Autodesk Inventor part; units mm, degrees
ref_plane "YZ Plane" through (0, 0, 0) normal (1, 0, 0) x (0, 1, 0)
ref_plane "XZ Plane" through (0, 0, 0) normal (0, 1, 0) x (-1, 0, 0)
ref_plane "XY Plane" through (0, 0, 0) normal (0, 0, 1) x (1, 0, 0)
sketch "Sketch1" plane through (0, 0, 0) normal (0, 1, 0) x (-1, 0, 0)
  line L0 (0, 0) -> (-40, 0)
  line L1 (-40, 0) -> (-160, 10)
  line L2 (-160, 10) -> (-160, 15)
  line L3 (-160, 15) -> (0, 15)
  line L4 (0, 15) -> (0, 0)
  point P0 (-160, 12.5)
  dimension "d0" = 15
  dimension "d1" = 40
  dimension "d2" = 5
  dimension "d3" = 120
extrude "Extrusion1" add sketch "Sketch1" along normal blind 16
sketch "Sketch2" plane through (0, 0, 15) normal (0, 0, 1) x (1, 0, 0)
  circle A0 centre (152.5, 8) radius 2.286
  circle A1 centre (47.5, 8) radius 2.286
  line L0 (160, 0) -> (160, 16)
  point P0 (0, 0)
  point P1 (160, 8)
  dimension "d6" = 4.572
  dimension "d7" = 7.5
  dimension "d8" = 105
extrude "Extrusion2" cut sketch "Sketch2" against normal blind 20
sketch "Sketch3" plane through (40, 0, 0) normal (0, 0, -1) x (-1, 0, 0)
  circle A0 centre (-112.5, 8) radius 2.286
  circle A1 centre (-112.5, 8) radius 6
  circle A2 centre (-7.5, 8) radius 2.286
  circle A3 centre (-7.5, 8) radius 6
  point P0 (40, 0)
  dimension "d11" = 12
extrude "Extrusion3" cut sketch "Sketch3" against normal up to surface (10 mm away)
sketch "Sketch4" plane through (40, 0, 0) normal (0, 0, -1) x (-1, 0, 0)
  line L0 (40, 0) -> (40, 16)
  line L1 (40, 0) -> (40, 16)
  line L2 (40, 16) -> (40, 26.5)
  line L3 (40, 26.5) -> (0, 26.5)
  line L4 (0, 26.5) -> (0, 16)
  line L5 (0, 0) -> (0, 16)
  line L6 (0, 0) -> (40, 0)
  line L7 (40, 0) -> (40, 16)
  line L8 (0, 16) -> (40, 16)
  point P0 (40, 8)
  dimension "d14" = 18.5
extrude "Extrusion4" add sketch "Sketch4" against normal up to surface (15 mm away) contours L8 L4 L3 L2
sketch "Sketch5" plane through (40, 0, 0) normal (0, 0, -1) x (-1, 0, 0)
  line L0 (40, 0) -> (-120, 0)
  line L1 (2, 0) -> (2, 13.8)
  line L2 (2, 13.8) -> (40, 13.8)
  line L3 (40, 0) -> (40, 26.5)
  line L4 (40, 26.5) -> (0, 26.5)
  line L5 (0, 26.5) -> (0, 16)
  dimension "d17" = 12.7
  dimension "d18" = 2
extrude "Extrusion5" cut sketch "Sketch5" against normal through all
sketch "Sketch6" plane through (40, 0, 15) normal (0, 0, -1) x (-1, 0, 0)
  line L0 (40, 13.8) -> (40, 26.5)
  line L1 (2, 13.8) -> (2, 0)
  line L2 (40, 13.8) -> (2, 0)
  line L3 (2, 13.8) -> (40, 13.8)
  point P0 (40, 0)
extrude "Extrusion6" add sketch "Sketch6" along normal blind 3
chamfer "Chamfer1" distance 3 angle 45 3 edges at (38, 6.9, 12) (38, 13.8, 6) (19, 13.8, 12)
sketch "Sketch7" plane through (160, 0, 15) normal (0, 0, 1) x (1, 0, 0)
  line L0 (-120, 26.5) -> (-120, 16)
  line L1 (-120, 26.5) -> (-85, 16)
  line L2 (-120, 16) -> (0, 16)
  point P0 (-160, 0)
  dimension "d29" = 35
extrude "Extrusion7" add sketch "Sketch7" against normal up to surface surface through (160, 0, 10) normal (0.0830455, 0, -0.9965458)
sketch "Sketch9" plane through (160, 0, 15) normal (0, 0, 1) x (1, 0, 0)
  circle A0 centre (-140, 21.15) radius 2.794
  circle A1 centre (-155, 21.15) radius 2.794
  line L0 (-160, 13.8) -> (-160, 26.5)
  point P0 (-160, 0)
  point P1 (-160, 15.8)
  point P2 (-160, 21.15)
  dimension "d32" = 5.588
  dimension "d33" = 15
  dimension "d34" = 5
extrude "Extrusion8" cut sketch "Sketch9" against normal through all
properties part number "Fan_side_mount"
For this review, take the finished solid that the model builds, in its own axes (mm). A direction names the side the tool comes from. Coordinates: 2 decimals unless noted, no trailing zeros. Order: outer loops, then holes, each group sorted by start corner. A loop starts at its lowest first (then second) coordinate and runs counter-clockwise, first axis right, second up. Notation, with made-up numbers: (-12.5, 31) -> (42.5, 31) arc R24 ccw to (42.5, 46) -> close; hole circle Ø9 at (59, 7). An arc over 180 degrees is marked (long way). Return JSON: item names as keys, results as strings.
1. We need section C-C on x = 70.5. Write out the cut boundary in (y, z).
Answer block:
{"outline": "(0, 2.54) -> (17.35, 2.54) -> (17.35, 15) -> (0, 15) -> close"}
2. The part is to be moulded in two halves that separate along Y. For faces 1 (the cylindrical face through (150.216, 8.101, 12.535)), 2 (the flat face through (86, 0, 9)), 3 (the flat face through (37, 5, 10)), 4 (the cylindrical face through (146.96, 5.7, 9.55)), say which applies: +Y half, -Y half, draft (parallel to the pull), parting line (faces both ways), or undercut.
Answer block:
{"face 1": "undercut", "face 2": "-Y half", "face 3": "draft", "face 4": "undercut"}
3. For line 1 (Y direction, x = 152.5, z = 11.2); line 2 (Y direction, x = 86, z = 10); line 3 (Y direction, x = 5, z = 12.25), list the stretches that pass through material, from the lowest coordinate up. Write a range as from..to.
Answer block:
{"line 1": "0..5.71, 10.29..16", "line 2": "0..16", "line 3": "11.98..18.36, 23.94..26.5"}
4. We need section D-D on y = 8. Write out the cut boundary in (x, z) (3 decimals), and give its area (3 significant figures).
Answer block:
{"outline": "(15.971, 12) -> (35, 12) -> (38, 9) -> (38, 0) -> (40, 0) -> (41.5, 0.125) -> (41.5, 10) -> (45.214, 10) -> (45.214, 15) -> (15.971, 15) -> close; (49.786, 10) -> (53.5, 10) -> (53.5, 1.125) -> (146.5, 8.875) -> (146.5, 10) -> (150.214, 10) -> (150.214, 15) -> (49.786, 15) -> close; (154.786, 10) -> (158.5, 10) -> (158.5, 9.875) -> (160, 10) -> (160, 15) -> (154.786, 15) -> close", "area": "1,130 mm²"}
5. We need section A-A on x = 5. Write out the cut boundary in (y, z), and give its area (3 significant figures).
Answer block:
{"outline": "(11.98, 10.82) -> (13.8, 9) -> (13.8, 0) -> (18.36, 0) -> (18.36, 15) -> (11.98, 15) -> close; (23.94, 0) -> (26.5, 0) -> (26.5, 15) -> (23.94, 15) -> close", "area": "116 mm²"}
6. Machinability: for faces 5 (the cylindrical face through (41.96, 5.7, 4.99)), 6 (the flat face through (25, 7, 12)), 7 (the flat face through (57.255, 21.323, 7.605)), which of the approach directions +Z, -Z, +X, -X, +Y, -Y give a long, thin tool a straight path to every point of the face, cutting with its end or side? Answer none if there is none.
Answer block:
{"face 5": "-Z", "face 6": "-Z, -X, -Y", "face 7": "+Z, -Z, +X, +Y"}
7. We need section B-B on y = 21.15. Write out the cut boundary in (x, z).
Answer block:
{"outline": "(0, 0) -> (2.21, 0) -> (2.21, 15) -> (0, 15) -> close; (7.79, 0) -> (17.21, 0) -> (17.21, 15) -> (7.79, 15) -> close; (22.79, 0) -> (40, 0) -> (57.83, 1.49) -> (57.83, 15) -> (22.79, 15) -> close"}
8. For pin 1 Ø9.5 at (x, y) = (152.5, 8) entering from -Z; pin 2 Ø2 at (x, z) = (43.5, 8) entering from +Y; pin 3 Ø1 at (x, z) = (88.5, 7.5) entering from +Y, all flat-tipped, find the tip position at first contact; note any pin that passes through.
Answer block:
{"pin 1": "z = 10", "pin 2": "y = 25.75", "pin 3": "y = 16"}
